```python
from build123d import *

# Parameters (mm, degrees)
BOSS_EXTRUDE1_DEPTH = 2.54
BOSS_EXTRUDE2_DEPTH = 1.016
SKETCH6_R           = 0.635
CUT_EXTRUDE1_DEPTH  = 2.54


with BuildPart() as part:
    # Sketch1 → Boss-Extrude1 (new body)
    with BuildSketch(Plane(origin=(0, 0, 0), x_dir=(0, 0, -1), z_dir=(1, 0, 0))):
        with BuildLine():
            Line((0.380788543, -13.474691937), (0.605560313, -6.731))
            Line((0.605560313, -6.731), (0.380788543, 0.012691937))
            ThreePointArc((0.380788543, 0.012691937), (0.2648824, 0.273858201), (0, 0.381))
            Line((0, 0.381), (-4.833515176, 0.381))
            ThreePointArc((-4.833515176, 0.381), (-5.098397576, 0.273858201), (-5.214303719, 0.012691937))
            Line((-5.214303719, 0.012691937), (-5.439075489, -6.731))
            Line((-5.439075489, -6.731), (-5.214303719, -13.474691937))
            ThreePointArc((-5.214303719, -13.474691937), (-5.098397576, -13.735858201), (-4.833515176, -13.843))
            Line((-4.833515176, -13.843), (0, -13.843))
            ThreePointArc((0, -13.843), (0.2648824, -13.735858201), (0.380788543, -13.474691937))
        make_face()
    extrude(amount=BOSS_EXTRUDE1_DEPTH)

    # Sketch5 → Boss-Extrude2 (add)
    with BuildSketch(Plane.ZY):
        with BuildLine():
            Line((0.130757588, -10.287), (4.702757588, -10.287))
            ThreePointArc((4.702757588, -10.287), (4.88236271, -10.212605122), (4.956757588, -10.033))
            Line((4.956757588, -10.033), (4.956757588, -3.429))
            ThreePointArc((4.956757588, -3.429), (4.88236271, -3.249394878), (4.702757588, -3.175))
            Line((4.702757588, -3.175), (0.130757588, -3.175))
            ThreePointArc((0.130757588, -3.175), (-0.048847535, -3.249394878), (-0.123242412, -3.429))
            Line((-0.123242412, -3.429), (-0.123242412, -10.033))
            ThreePointArc((-0.123242412, -10.033), (-0.048847535, -10.212605122), (0.130757588, -10.287))
        make_face()
    extrude(amount=BOSS_EXTRUDE2_DEPTH)

    # Sketch6 → Cut-Extrude1 (cut)
    with BuildSketch(Plane.ZY.offset(1.016)):
        with Locations((2.416757588, -5.461)):
            Circle(SKETCH6_R)
        with Locations((2.416757588, -8.001)):
            Circle(SKETCH6_R)
    extrude(amount=-CUT_EXTRUDE1_DEPTH, mode=Mode.SUBTRACT)


solid = part.part
```
Geometry check sheet. Reference: the model listing, model coordinates, mm. A direction names the side the tool comes from. Give positions to 0.01 mm unless a question says otherwise; leave off trailing zeros. Order: outer loops, then holes, each group sorted by start corner. A loop starts at its lowest first (then second) coordinate and runs counter-clockwise, first axis right, second up.
1. Section check D-D, the plane x = 1.3. Enter the section's corners in (y, z) (3 decimals), and give its area (3 significant figures).
2. Access from +Z, -Z, +X, -X, +Y, -Y to the whole of each face (thin tool, end or side, straight path). Record for faces 1 (the face through (-0.5, -3.175, 2.4)), 2 (the face through (-0.5, -10.287, 2.4)), 3 (the face through (1, -13.843, 2)), 4 (the face through (0.24, -6.08, 2.28)), 5 (the face through (1, 0.381, 2)).
3. Section check C-C, the plane y = -9. Enter the section's corners in (x, z), and give its area (3 significant figures).
4. Thickness scan on L1, parallel to Y at x = -0.4, z = 2.5 (3 decimals); L2, parallel to Y at x = 0.3, z = 2; L3, parallel to Y at x = -0.8, z = 1.5 (3 decimals). Record the ranges inside material, lowest first.
5. Section check B-B, the plane x = 2. Enter the section's corners in (y, z).
6. Section check A-A, the plane z = 4.25. Enter the section's corners in (x, y) (3 decimals).
7. Release check for a two-part mould opening along Z. For faces 6 (the face through (-0.5, -6.7, -0.123)), 7 (the face through (-1.016, -7, 2)), 8 (the face through (1.524, -5.5, 2.4)), 9 (the face through (-0.5, -6.8, 4.957)) record: pulls with the +Z half, pulls with the -Z half, needs draft (parallel to the pull), parting line crosses it, or undercut.
8. Gauge pin test, flat ends, axial feed: pin 1 Ø0.6 at (y, z) = (-5.5, 2.5) entering from -X; pin 2 Ø1.5 at (x, y) = (0.5, -9.5) entering from +Z; pin 3 Ø0.5 at (x, y) = (-0.5, -7.5) entering from +Z; pin 4 Ø1.1 at (x, z) = (-0.5, 2.5) entering from -Y. Record the tip position at first contact, or that the pin passes through.
Values follow:
1. outline: (-13.843, 0) arc R0.381 ccw to (-13.475, -0.381) - (-6.731, -0.606) - (0.013, -0.381) arc R0.381 ccw to (0.381, 0) - (0.381, 4.834) arc R0.381 ccw to (0.013, 5.214) - (-6.731, 5.439) - (-13.475, 5.214) arc R0.381 ccw to (-13.843, 4.834) - close; hole circle Ø1.27 at (-8.001, 2.417); hole circle Ø1.27 at (-5.461, 2.417)
1. area: 80.0 mm2
2. face 1: +Z, -Z, -X, +Y
2. face 2: +Z, -Z, -X, -Y
2. face 3: +Z, -Z, +X, -X, -Y
2. face 4: -X
2. face 5: +Z, -Z, +X, -X, +Y
3. outline: (-1.02, -0.12) - (0, -0.12) - (0, -0.53) - (2.54, -0.53) - (2.54, 5.36) - (0, 5.36) - (0, 4.96) - (-1.02, 4.96) - close
3. area: 20.1 mm2
4. L1: y = -10.287 to -8.631, -7.371 to -6.091, -4.831 to -3.175
4. L2: y = -13.84 to -8.48, -7.52 to -5.94, -4.98 to 0.38
4. L3: y = -10.287 to -3.175
5. outline: (-13.84, 0) arc R0.38 ccw to (-13.47, -0.38) - (-6.73, -0.61) - (0.01, -0.38) arc R0.38 ccw to (0.38, 0) - (0.38, 4.83) arc R0.38 ccw to (0.01, 5.21) - (-6.73, 5.44) - (-13.47, 5.21) arc R0.38 ccw to (-13.84, 4.83) - close
6. outline: (-1.016, -10.287) - (0, -10.287) - (0, -13.843) - (2.54, -13.843) - (2.54, 0.381) - (0, 0.381) - (0, -3.175) - (-1.016, -3.175) - close
7. face 6: pulls with the -Z half
7. face 7: needs draft
7. face 8: undercut
7. face 9: pulls with the +Z half
8. pin 1: stops at x = 1.52
8. pin 2: stops at z = 5.37
8. pin 3: stops at z = 4.96
8. pin 4: stops at y = -13.84
